Design review of the part built by this model. Coordinates are the model's own, in mm. Give positions to 0.01 mm unless a question says otherwise; leave off trailing zeros. Order: outer loops, then holes, each group sorted by start corner. A loop starts at its lowest first (then second) coordinate and runs counter-clockwise, first axis right, second up. Notation, with made-up numbers: (26.5, 13) -> (35.5, 13) arc R22 ccw to (35.5, 37) -> close; hole circle Ø11 at (27, -8). An arc over 180 degrees is marked (long way). Return JSON: item names as keys, results as strings.
```python
from build123d import *

# Parameters (mm, degrees)
BOSS_EXTRUDE1_DEPTH = 2.8956


with BuildPart() as part:
    # Sketch1 → Boss-Extrude1 (new body)
    with BuildSketch(Plane(origin=(0, 0, 0), x_dir=(1, 0, 0), z_dir=(0, 1, 0))):
        with BuildLine():
            Line((21.59, 1.2446), (25.393976036, 1.2446))
            add(Edge.make_bspline(
                [(25.393976036, 1.2446), (25.305125525, 10.422131382), (23.943355437, 19.0754)],
                knots=[4.73416848, 4.73416848, 4.73416848, 5.052697334, 5.052697334, 5.052697334], degree=2, weights=[1, 0.987344206, 1]))
            Line((23.943355437, 19.0754), (19.930240776, 19.0754))
            Line((19.930240776, 19.0754), (19.930240776, 21.5646))
            Line((19.930240776, 21.5646), (23.522368768, 21.5646))
            add(Edge.make_bspline(
                [(23.522368768, 21.5646), (0, 151.457597173), (-23.522368768, 21.5646)],
                knots=[5.099304053, 5.099304053, 5.099304053, 7.467066561, 7.467066561, 7.467066561], degree=2, weights=[1, 0.377333333, 1]))
            Line((-23.522368768, 21.5646), (-19.930240776, 21.5646))
            Line((-19.930240776, 21.5646), (-19.930240776, 19.0754))
            Line((-19.930240776, 19.0754), (-23.943355437, 19.0754))
            add(Edge.make_bspline(
                [(-23.943355437, 19.0754), (-25.305125525, 10.422131382), (-25.393976036, 1.2446)],
                knots=[1.230487974, 1.230487974, 1.230487974, 1.549016827, 1.549016827, 1.549016827], degree=2, weights=[1, 0.987344206, 1]))
            Line((-25.393976036, 1.2446), (-21.59, 1.2446))
            Line((-21.59, 1.2446), (-21.59, -1.2446))
            Line((-21.59, -1.2446), (-25.393976036, -1.2446))
            add(Edge.make_bspline(
                [(-25.393976036, -1.2446), (-25.305125525, -10.422131382), (-23.943355437, -19.0754)],
                knots=[1.592575826, 1.592575826, 1.592575826, 1.91110468, 1.91110468, 1.91110468], degree=2, weights=[1, 0.987344206, 1]))
            Line((-23.943355437, -19.0754), (-19.930240776, -19.0754))
            Line((-19.930240776, -19.0754), (-19.930240776, -21.5646))
            Line((-19.930240776, -21.5646), (-23.522368768, -21.5646))
            add(Edge.make_bspline(
                [(-23.522368768, -21.5646), (-22.395811131, -27.785569894), (-20.658836503, -33.249220312)],
                knots=[1.957711399, 1.957711399, 1.957711399, 2.191722412, 2.191722412, 2.191722412], degree=2, weights=[1, 0.993162662, 1]))
            Line((-20.658836503, -33.249220312), (-40.656934115, -75.189915873))
            ThreePointArc((-40.656934115, -75.189915873), (-40.089838211, -78.146952179), (-37.097948163, -78.484969079))
            Line((-37.097948163, -78.484969079), (-8.029094451, -54.219568092))
            add(Edge.make_bspline(
                [(-8.029094451, -54.219568092), (-4.724069079, -56.697277371), (-1.2446, -57.081350193)],
                knots=[2.819970364, 2.819970364, 2.819970364, 3.092573024, 3.092573024, 3.092573024], degree=2, weights=[1, 0.990725346, 1]))
            Line((-1.2446, -57.081350193), (-1.2446, -53.975))
            Line((-1.2446, -53.975), (-1.2446, -50.644928526))
            add(Edge.make_bspline(
                [(-1.2446, -50.644928526), (-1.592566722, -50.559021859), (-2.797472305, -50.153191319), (-5.318112389, -48.514264833), (-8.117471478, -45.20633596), (-9.696301311, -42.637606864), (-10.124198394, -41.884600001)],
                knots=[-3.032554281, -3.032554281, -3.032554281, -3.032554281, -2.945243113, -2.748893572, -2.552544031, -2.478028469, -2.478028469, -2.478028469, -2.478028469], degree=3))
            Line((-10.124198394, -41.884600001), (-14.613224312, -41.884600001))
            Line((-14.613224312, -41.884600001), (-14.613224312, -39.395400001))
            Line((-14.613224312, -39.395400001), (-11.431305901, -39.395400001))
            add(Edge.make_bspline(
                [(-11.431305901, -39.395400001), (-11.677149239, -38.889598832), (-12.987812642, -36.070874709), (-15.148196965, -30.166196648), (-18.099752632, -17.775460251), (-19.683498245, 0), (-18.099752632, 17.775460251), (-15.148196965, 30.166196648), (-12.987812642, 36.070874709), (-11.677149239, 38.889598832), (-11.431305901, 39.395400001)],
                knots=[-2.400745736, -2.400745736, -2.400745736, -2.400745736, -2.35619449, -2.159844949, -1.963495408, -1.570796327, -1.178097245, -0.981747704, -0.785398163, -0.740846918, -0.740846918, -0.740846918, -0.740846918], degree=3))
            Line((-11.431305901, 39.395400001), (-14.613224312, 39.395400001))
            Line((-14.613224312, 39.395400001), (-14.613224312, 41.884600001))
            Line((-14.613224312, 41.884600001), (-10.124198394, 41.884600001))
            add(Edge.make_bspline(
                [(-10.124198394, 41.884600001), (-9.696301311, 42.637606864), (-8.117471478, 45.20633596), (-5.318112389, 48.514264833), (-2.797472305, 50.153191319), (-1.592566722, 50.559021859), (-1.2446, 50.644928526)],
                knots=[-0.663564185, -0.663564185, -0.663564185, -0.663564185, -0.589048623, -0.392699082, -0.196349541, -0.109038372, -0.109038372, -0.109038372, -0.109038372], degree=3))
            Line((-1.2446, 50.644928526), (-1.2446, 53.975))
            Line((-1.2446, 53.975), (1.2446, 53.975))
            Line((1.2446, 53.975), (1.2446, 50.644928526))
            add(Edge.make_bspline(
                [(10.124198394, 41.884600001), (9.696301311, 42.637606864), (8.117471478, 45.20633596), (5.318112389, 48.514264833), (2.797472305, 50.153191319), (1.592566722, 50.559021859), (1.2446, 50.644928526)],
                knots=[-0.663564185, -0.663564185, -0.663564185, -0.663564185, -0.589048623, -0.392699082, -0.196349541, -0.109038372, -0.109038372, -0.109038372, -0.109038372], degree=3))
            Line((10.124198394, 41.884600001), (14.613224312, 41.884600001))
            Line((14.613224312, 41.884600001), (14.613224312, 39.395400001))
            Line((14.613224312, 39.395400001), (11.431305901, 39.395400001))
            add(Edge.make_bspline(
                [(11.431305901, -39.395400001), (11.677149239, -38.889598832), (12.987812642, -36.070874709), (15.148196965, -30.166196648), (18.099752632, -17.775460251), (19.683498245, 0), (18.099752632, 17.775460251), (15.148196965, 30.166196648), (12.987812642, 36.070874709), (11.677149239, 38.889598832), (11.431305901, 39.395400001)],
                knots=[-2.400745736, -2.400745736, -2.400745736, -2.400745736, -2.35619449, -2.159844949, -1.963495408, -1.570796327, -1.178097245, -0.981747704, -0.785398163, -0.740846918, -0.740846918, -0.740846918, -0.740846918], degree=3))
            Line((11.431305901, -39.395400001), (14.613224312, -39.395400001))
            Line((14.613224312, -39.395400001), (14.613224312, -41.884600001))
            Line((14.613224312, -41.884600001), (10.124198394, -41.884600001))
            add(Edge.make_bspline(
                [(1.2446, -50.644928526), (1.592566722, -50.559021859), (2.797472305, -50.153191319), (5.318112389, -48.514264833), (8.117471478, -45.20633596), (9.696301311, -42.637606864), (10.124198394, -41.884600001)],
                knots=[-3.032554281, -3.032554281, -3.032554281, -3.032554281, -2.945243113, -2.748893572, -2.552544031, -2.478028469, -2.478028469, -2.478028469, -2.478028469], degree=3))
            Line((1.2446, -50.644928526), (1.2446, -53.975))
            Line((1.2446, -53.975), (1.2446, -57.081350193))
            add(Edge.make_bspline(
                [(1.2446, -57.081350193), (4.724069079, -56.697277371), (8.029094451, -54.219568092)],
                knots=[3.190612283, 3.190612283, 3.190612283, 3.463214943, 3.463214943, 3.463214943], degree=2, weights=[1, 0.990725346, 1]))
            Line((8.029094451, -54.219568092), (37.097948163, -78.484969079))
            ThreePointArc((37.097948163, -78.484969079), (40.089838211, -78.146952179), (40.656934115, -75.189915873))
            Line((40.656934115, -75.189915873), (20.658836503, -33.249220312))
            add(Edge.make_bspline(
                [(20.658836503, -33.249220312), (22.395811131, -27.785569894), (23.522368768, -21.5646)],
                knots=[4.091462895, 4.091462895, 4.091462895, 4.325473908, 4.325473908, 4.325473908], degree=2, weights=[1, 0.993162662, 1]))
            Line((23.522368768, -21.5646), (19.930240776, -21.5646))
            Line((19.930240776, -21.5646), (19.930240776, -19.0754))
            Line((19.930240776, -19.0754), (23.943355437, -19.0754))
            add(Edge.make_bspline(
                [(23.943355437, -19.0754), (25.305125525, -10.422131382), (25.393976036, -1.2446)],
                knots=[4.372080627, 4.372080627, 4.372080627, 4.690609481, 4.690609481, 4.690609481], degree=2, weights=[1, 0.987344206, 1]))
            Line((25.393976036, -1.2446), (21.59, -1.2446))
            Line((21.59, -1.2446), (21.59, 1.2446))
        make_face()
    extrude(amount=BOSS_EXTRUDE1_DEPTH)


solid = part.part
```
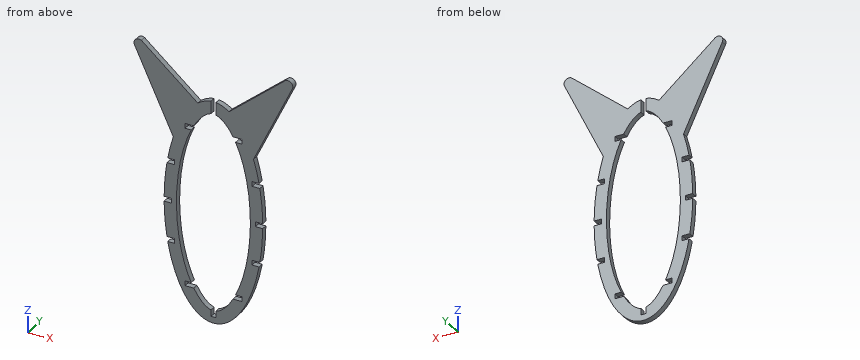
Item 1: Add section A-A (z = 59). Give the boundary of the cut face in (x, y).
Result set:
{"outline": "(-32.94, 0) -> (-13.76, 0) -> (-13.76, 2.9) -> (-32.94, 2.9) -> close; (13.76, 0) -> (32.94, 0) -> (32.94, 2.9) -> (13.76, 2.9) -> close"}
Item 2: Add section C-C (x = -31). Give the boundary of the cut face in (y, z).
Result set:
{"outline": "(0, 54.94) -> (2.9, 54.94) -> (2.9, 73.39) -> (0, 73.39) -> close"}
Item 3: Wall thickness on L1, parallel to X at y = 2.1, z = 2; L2, parallel to Z at x = 6, y = 1; L3, parallel to X at y = 1.25, z = -7: over which ranges is each line inside the solid? List them lowest first. Write a range as [from, to].
Result set:
{"L1": "x = [-25.38, -19.03], [19.03, 25.38]", "L2": "z = [-55.53, -47.56], [47.56, 55.53]", "L3": "x = [-25.21, -18.85], [18.85, 25.21]"}
Item 4: Add section B-B (x = 30). Give the boundary of the cut face in (y, z).
Result set:
{"outline": "(0, 52.84) -> (2.9, 52.84) -> (2.9, 72.56) -> (0, 72.56) -> close"}
Item 5: For pin 1 (0.9 mm diameter, centred on x = 12.5, y = 1, fed in from +Z); pin 2 (1 mm diameter, centred on x = 14, z = -26.5, fed in from +Y); pin 3 (1.5 mm diameter, centred on y = 1.5, z = -30, fed in from +X); pin 4 (0.9 mm diameter, centred on x = -13, y = 1, fed in from +Z), all flat-tipped, find the tip position at first contact; note any pin that passes through.
Result set:
{"pin 1": "stops at z = 58.33", "pin 2": "passes through", "pin 3": "stops at x = 21.82", "pin 4": "stops at z = 58.74"}
